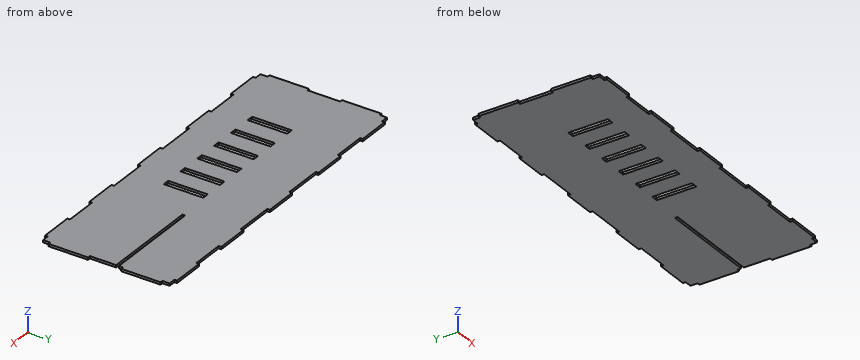
```python
from build123d import *

# Parameters (mm, degrees)
SKETCH_1_W          = 500
SKETCH_1_H          = 200
EXTRUDE_1_DEPTH     = 3.6
SKETCH_3_W          = 4
SKETCH_3_H          = 50
CUT_EXTRUDE_2_DEPTH = 3.6
SKETCH_4_W          = 56.911563003
SKETCH_4_H          = 4
SKETCH_4_W_2        = 50
SKETCH_4_W_3        = 60
SKETCH_4_W_4        = 57.96169575
CUT_EXTRUDE_3_DEPTH = 10
SKETCH_5_W          = 10
SKETCH_5_H          = 60
CUT_EXTRUDE_4_DEPTH = 270.282305397
SKETCH_6_W          = 194.899640321
SKETCH_6_H          = 4
CUT_EXTRUDE_5_DEPTH = 270.282305397


with BuildPart() as part:
    # 草图1 → 凸台-拉伸1 (new body)
    with BuildSketch(Plane.XY):
        Rectangle(SKETCH_1_W, SKETCH_1_H)
    extrude(amount=EXTRUDE_1_DEPTH)

    # 草图3 → 切除-拉伸2 (cut)
    with BuildSketch(Plane.XY.offset(3.6)):
        with Locations((-248, 0)):
            Rectangle(SKETCH_3_W, SKETCH_3_H)
        with Locations((-248, 110)):
            Rectangle(SKETCH_3_W, SKETCH_3_H)
        with Locations((-248, -110)):
            Rectangle(SKETCH_3_W, SKETCH_3_H)
        with Locations((248, 110)):
            Rectangle(SKETCH_3_W, SKETCH_3_H)
        with Locations((248, 0)):
            Rectangle(SKETCH_3_W, SKETCH_3_H)
        with Locations((248, -110)):
            Rectangle(SKETCH_3_W, SKETCH_3_H)
    extrude(amount=-CUT_EXTRUDE_2_DEPTH, mode=Mode.SUBTRACT)

    # 草图4 → 切除-拉伸3 (cut)
    with BuildSketch(Plane.XY.offset(3.6)):
        with Locations((-263.455781502, -98)):
            Rectangle(SKETCH_4_W, SKETCH_4_H)
        with Locations((-160, -98)):
            Rectangle(SKETCH_4_W_2, SKETCH_4_H)
        with Locations((-55, -98)):
            Rectangle(SKETCH_4_W_3, SKETCH_4_H)
        with Locations((55, -98)):
            Rectangle(SKETCH_4_W_3, SKETCH_4_H)
        with Locations((160, -98)):
            Rectangle(SKETCH_4_W_2, SKETCH_4_H)
        with Locations((263.980847875, -98)):
            Rectangle(SKETCH_4_W_4, SKETCH_4_H)
        with Locations((263.980847875, 98)):
            Rectangle(SKETCH_4_W_4, SKETCH_4_H)
        with Locations((160, 98)):
            Rectangle(SKETCH_4_W_2, SKETCH_4_H)
        with Locations((55, 98)):
            Rectangle(SKETCH_4_W_3, SKETCH_4_H)
        with Locations((-55, 98)):
            Rectangle(SKETCH_4_W_3, SKETCH_4_H)
        with Locations((-160, 98)):
            Rectangle(SKETCH_4_W_2, SKETCH_4_H)
        with Locations((-263.455781502, 98)):
            Rectangle(SKETCH_4_W, SKETCH_4_H)
    extrude(amount=-CUT_EXTRUDE_3_DEPTH, mode=Mode.SUBTRACT)

    # 草图5 → 切除-拉伸4 (cut, through all)
    with BuildSketch(Plane.XY.offset(3.6)):
        with Locations((-148, -16.237417244)):
            Rectangle(SKETCH_5_W, SKETCH_5_H)
        with Locations((-110, -16.237417244)):
            Rectangle(SKETCH_5_W, SKETCH_5_H)
        with Locations((-72, -16.237417244)):
            Rectangle(SKETCH_5_W, SKETCH_5_H)
        with Locations((-34, -16.237417244)):
            Rectangle(SKETCH_5_W, SKETCH_5_H)
        with Locations((4, -16.237417244)):
            Rectangle(SKETCH_5_W, SKETCH_5_H)
        with Locations((42, -16.237417244)):
            Rectangle(SKETCH_5_W, SKETCH_5_H)
    extrude(amount=-CUT_EXTRUDE_4_DEPTH, mode=Mode.SUBTRACT)

    # 草图6 → 切除-拉伸5 (cut, through all)
    with BuildSketch(Plane.XY.offset(3.6)):
        with Locations((193.44982016, 17)):
            Rectangle(SKETCH_6_W, SKETCH_6_H)
    extrude(amount=-CUT_EXTRUDE_5_DEPTH, mode=Mode.SUBTRACT)


solid = part.part
```
Could you check a few things on this model? Use its own coordinates, in mm. Give positions to 0.01 mm unless a question says otherwise; leave off trailing zeros. Loops run counter-clockwise (first coordinate to the right, second up) from the corner with the lowest first, then second, coordinate; pieces in that order, holes last. Notation, with made-up numbers: (48, 66) - (68, 66) arc R16 cw to (68, 96) - close; hole circle Ø5 at (6, 89.5). An arc over 180 degrees is marked (long way). Answer in a Markdown table with one row per item. Add a question column.
Q1. For pin 1 (1.1 mm diameter, centred on y = 99, z = 1.5, fed in from -X); pin 2 (1.8 mm diameter, centred on y = -1.5, z = 2, fed in from +X); pin 3 (1.8 mm diameter, centred on y = 97.5, z = 2, fed in from +X), each with a flat end and sliding along its axis, tell me the tip position at first contact or that it passes through.
Q2. Please list where these lines run through material, in increasing order: L1, parallel to Y at x = -30.5, z = 3.3; L2, parallel to Y at x = 179.5, z = 2.9; L3, parallel to X at y = -88.5, z = 0.9. Write a range as from..to.
Q3. If we section it at C-C (z = 2.25): State how many separate pieces and enclosed holes the cut face has, plus the area to 3 significant figures.
Q4. If we section it at B-B (y = -35): List the corners of the cut face in (x, z) for me, plus the area to 3 significant figures.
Q5. If we section it at A-A (x = 207.5): List the corners of the cut face in (y, z) for me.
Q6. If we section it at D-D (y = -11.5): List the corners of the cut face in (x, z) for me, plus the area to 3 significant figures.
The answers:
| question | item | result |
|---|---|---|
| 1 | pin 1 | stops at x = -235 |
| 1 | pin 2 | stops at x = 246 |
| 1 | pin 3 | stops at x = 235 |
| 2 | L1 | y = -96..-46.24, 13.76..96 |
| 2 | L2 | y = -96..15, 19..96 |
| 2 | L3 | x = -246..246 |
| 3 | separate pieces | 1 |
| 3 | enclosed holes | 6 |
| 3 | area | 93,200 mm^2 |
| 4 | outline | (-250, 0) - (-153, 0) - (-153, 3.6) - (-250, 3.6) - close; (-143, 0) - (-115, 0) - (-115, 3.6) - (-143, 3.6) - close; (-105, 0) - (-77, 0) - (-77, 3.6) - (-105, 3.6) - close; (-67, 0) - (-39, 0) - (-39, 3.6) - (-67, 3.6) - close; (-29, 0) - (-1, 0) - (-1, 3.6) - (-29, 3.6) - close; (9, 0) - (37, 0) - (37, 3.6) - (9, 3.6) - close; (47, 0) - (250, 0) - (250, 3.6) - (47, 3.6) - close |
| 4 | area | 1,580 mm^2 |
| 5 | outline | (-100, 0) - (15, 0) - (15, 3.6) - (-100, 3.6) - close; (19, 0) - (100, 0) - (100, 3.6) - (19, 3.6) - close |
| 6 | outline | (-246, 0) - (-153, 0) - (-153, 3.6) - (-246, 3.6) - close; (-143, 0) - (-115, 0) - (-115, 3.6) - (-143, 3.6) - close; (-105, 0) - (-77, 0) - (-77, 3.6) - (-105, 3.6) - close; (-67, 0) - (-39, 0) - (-39, 3.6) - (-67, 3.6) - close; (-29, 0) - (-1, 0) - (-1, 3.6) - (-29, 3.6) - close; (9, 0) - (37, 0) - (37, 3.6) - (9, 3.6) - close; (47, 0) - (246, 0) - (246, 3.6) - (47, 3.6) - close |
| 6 | area | 1,560 mm^2 |
